Part model, mm, in its own coordinate system. Face numbers are marked on the shaded views. Round coordinates to 2 decimals unless told otherwise and drop trailing zeros. Order: outer loops, then holes, each group sorted by start corner. A loop starts at its lowest first (then second) coordinate and runs counter-clockwise, first axis right, second up. Notation, with made-up numbers: M 76,-14.75 L 87,-14.75 A13 cw 87,-4.75 Z; hole C 52,-38.75 d3. An arc over 180 degrees is marked long. Write each question's results on one line, items separated by ' | '. Start each with the question number.
1. Drop a flat-ended pin along its axis: pin 1 Ø6 at (x, z) = (36, 1) entering from -Y. Give the stop position or say it passes through.
2. Band-saw the part on A-A, the plane x = 10. List the corners of the cut face in (y, z).
3. Probe L1, parallel to X at y = 83, z = 5.5; L2, parallel to Y at x = 7.5, z = 9.5; L3, parallel to X at y = 116.5, z = 8. List the from-to ranges inside material, lowest first. Write a range as [from, to].
4. Band-saw the part on B-B, the plane x = 22. List the corners of the cut face in (y, z), then the cut area to 3 significant figures.
5. Two-plate mould, pull along Y, no slides. Class the marked faces 1 and 2: +Y half, -Y half, draft (parallel to the pull), parting line (faces both ways), or undercut.
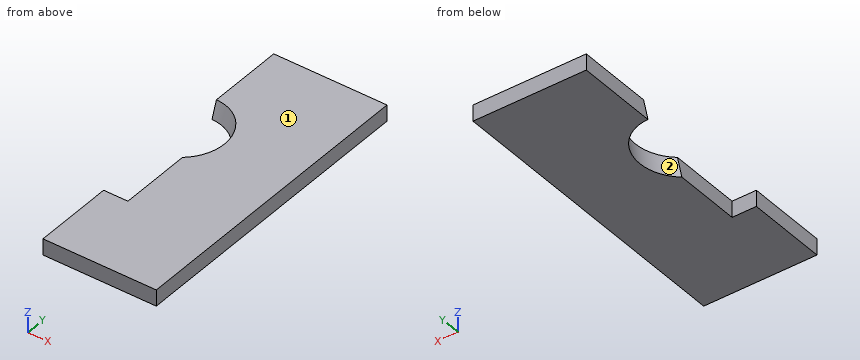
```python
from build123d import *

# Parameters (mm, degrees)
ESQUISSE1_W             = 70
ESQUISSE1_H             = 190
BOSS_EXTRU_1_DEPTH      = 10
ENL_V_MAT_EXTRU_1_DEPTH = 203.731349327
ESQUISSE3_W             = 15
ESQUISSE3_H             = 45
ENL_V_MAT_EXTRU_2_DEPTH = 203.731349327


with BuildPart() as part:
    # Esquisse1 → Boss.-Extru.1 (new body)
    with BuildSketch(Plane.XY):
        with Locations((35, 95)):
            Rectangle(ESQUISSE1_W, ESQUISSE1_H)
    extrude(amount=BOSS_EXTRU_1_DEPTH)

    # Esquisse2 → Enlèv. mat.-Extru.1 (cut, through all)
    with BuildSketch(Plane(origin=(0, 0, 0), x_dir=(1, 0, 0), z_dir=(0, -0.34202014332566943, -0.9396926207859081))):
        with BuildLine():
            Line((0, -80.778483455), (0, -130.778483455))
            ThreePointArc((0, -130.778483455), (25, -105.778483455), (0, -80.778483455))
        make_face()
    extrude(amount=-ENL_V_MAT_EXTRU_1_DEPTH, mode=Mode.SUBTRACT)

    # Esquisse3 → Enlèv. mat.-Extru.2 (cut, through all)
    with BuildSketch(Plane(origin=(0, 0, 0), x_dir=(-1, 0, 0), z_dir=(0, 0, -1))):
        with Locations((-7.5, 72.423257792)):
            Rectangle(ESQUISSE3_W, ESQUISSE3_H)
    extrude(amount=-ENL_V_MAT_EXTRU_2_DEPTH, mode=Mode.SUBTRACT)


solid = part.part
```
Solution:
1) pin 1: y = 0
2) outline: M 0,0 L 49.92,0 L 49.92,10 L 0,10 Z; M 136.95,0 L 190,0 L 190,10 L 140.59,10 Z
3) L1: [15, 70] | L2: [0, 49.92], [141.4, 190] | L3: [24.98, 70]
4) outline: M 0,0 L 99.93,0 L 103.57,10 L 0,10 Z; M 125.2,0 L 190,0 L 190,10 L 128.84,10 Z | area: 1,650 mm^2
5) face 1: draft | face 2: undercut
